from build123d import *

# Parameters (mm, degrees)
SKETCH1_R           = 2.5
BOSS_EXTRUDE3_DEPTH = 1.5
FILLET1_R           = 2.5
SKETCH3_R           = 10
SKETCH3_R_2         = 2.5
BOSS_EXTRUDE4_DEPTH = 7


with BuildPart() as part:
    # Sketch1 → Boss-Extrude3 (new body)
    with BuildSketch(Plane(origin=(0, 0, 0), x_dir=(0, 0, -1), z_dir=(1, 0, 0))):
        with BuildLine():
            Line((-34.72862652, 4.35), (-33.15, 4.35))
            Line((-33.15, 4.35), (-33.15, -4.35))
            Line((-33.15, -4.35), (-34.72862652, -4.35))
            ThreePointArc((-34.72862652, -4.35), (-24.748737342, -24.748737342), (-4.35, -34.72862652))
            Line((-4.35, -34.72862652), (-4.35, -33.15))
            Line((-4.35, -33.15), (4.35, -33.15))
            Line((4.35, -33.15), (4.35, -34.72862652))
            ThreePointArc((4.35, -34.72862652), (24.748737342, -24.748737342), (34.72862652, -4.35))
            Line((34.72862652, -4.35), (33.15, -4.35))
            Line((33.15, -4.35), (33.15, 4.35))
            Line((33.15, 4.35), (34.72862652, 4.35))
            ThreePointArc((34.72862652, 4.35), (24.748737342, 24.748737342), (4.35, 34.72862652))
            Line((4.35, 34.72862652), (4.35, 33.15))
            Line((4.35, 33.15), (-4.35, 33.15))
            Line((-4.35, 33.15), (-4.35, 34.72862652))
            ThreePointArc((-4.35, 34.72862652), (-24.748737342, 24.748737342), (-34.72862652, 4.35))
        make_face()
        Circle(SKETCH1_R, mode=Mode.SUBTRACT)
        with BuildLine():
            Line((9.270248109, 3.75), (27.243118397, 3.75))
            ThreePointArc((27.243118397, 3.75), (19.17641557, 19.71078603), (3, 27.335873866))
            Line((3, 27.335873866), (3, 9.539392014))
            ThreePointArc((3, 9.539392014), (6.783731432, 7.347175502), (9.270248109, 3.75))
        make_face(mode=Mode.SUBTRACT)
        with BuildLine():
            Line((-3, 9.539392014), (-3, 27.335873866))
            ThreePointArc((-3, 27.335873866), (-19.709993452, 19.177230199), (-27.407799985, 2.25))
            Line((-27.407799985, 2.25), (-9.743587635, 2.25))
            ThreePointArc((-9.743587635, 2.25), (-7.340542585, 6.790908228), (-3, 9.539392014))
        make_face(mode=Mode.SUBTRACT)
        with BuildLine():
            Line((9.743587635, -2.25), (27.407799985, -2.25))
            ThreePointArc((27.407799985, -2.25), (20.230473673, -18.627343744), (4.5, -27.129319933))
            Line((4.5, -27.129319933), (4.5, -8.93028555))
            ThreePointArc((4.5, -8.93028555), (7.866161766, -6.174422974), (9.743587635, -2.25))
        make_face(mode=Mode.SUBTRACT)
        with BuildLine():
            Line((-1.5, -9.886859967), (-1.5, -27.459060435))
            ThreePointArc((-1.5, -27.459060435), (-18.629857769, -20.22815858), (-27.243118397, -3.75))
            Line((-27.243118397, -3.75), (-9.270248109, -3.75))
            ThreePointArc((-9.270248109, -3.75), (-6.197969316, -7.847622338), (-1.5, -9.886859967))
        make_face(mode=Mode.SUBTRACT)
    extrude(amount=BOSS_EXTRUDE3_DEPTH)

    # Fillet1
    fillet1_edges = [part.edges().sort_by_distance(p)[0] for p in [
        (0.75, -9.886859967, 1.5),
        (0.75, -3.75, 9.270248109),
        (0.75, -3.75, 27.243118397),
        (0.75, -27.459060435, 1.5),
        (0.75, 27.335873866, 3),
        (0.75, 2.25, 27.407799985),
        (0.75, 2.25, 9.743587635),
        (0.75, 9.539392014, 3),
        (0.75, 3.75, -27.243118397),
        (0.75, 27.335873866, -3),
        (0.75, 9.539392014, -3),
        (0.75, 3.75, -9.270248109),
        (0.75, -2.25, -9.743587635),
        (0.75, -8.93028555, -4.5),
        (0.75, -27.129319933, -4.5),
        (0.75, -2.25, -27.407799985),
    ]]
    fillet(fillet1_edges, radius=FILLET1_R)

    # Sketch3 → Boss-Extrude4 (add)
    with BuildSketch(Plane(origin=(1.5, 0, 0), x_dir=(0, 0, -1), z_dir=(1, 0, 0))):
        with Locations(Location((0, 0, 0), (0, 0, 157.666317342))):
            Circle(SKETCH3_R)
        Circle(SKETCH3_R_2, mode=Mode.SUBTRACT)
    extrude(amount=BOSS_EXTRUDE4_DEPTH)


solid = part.part
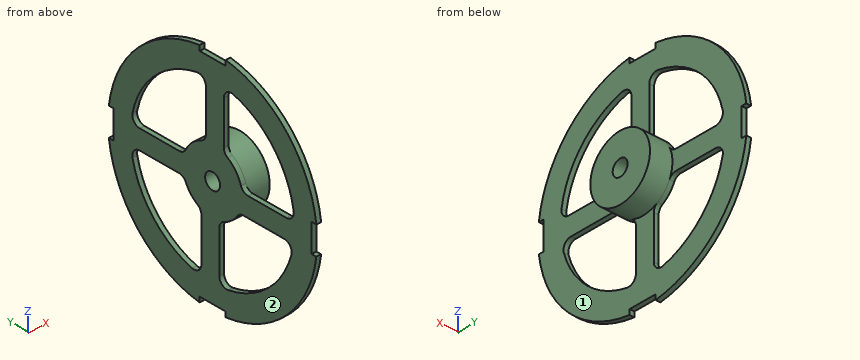
Geometry: final body of the model. Coordinates: model frame, mm. Face numbers are marked on the shaded views. A direction names the side the tool comes from. Coordinates: 2 decimals unless noted, no trailing zeros. Order: outer loops, then holes, each group sorted by start corner. A loop starts at its lowest first (then second) coordinate and runs counter-clockwise, first axis right, second up. Notation, with made-up numbers: (13, -38) - (51, -38) arc R21 ccw to (51, -2) - close; hole circle Ø3 at (36.25, 20.25). An arc over 180 degrees is marked (long way). Use one line per item in the form item = value.
1) Section D-D (z = -14). Return loops of the section in (x, y), then the cut area to 3 significant figures.
Solutions:
outline = (0, -32.08) - (1.5, -32.08) - (1.5, -23.67) - (0, -23.67) - close; (0, -2.25) - (1.5, -2.25) - (1.5, 3.75) - (0, 3.75) - close; (0, 23.67) - (1.5, 23.67) - (1.5, 32.08) - (0, 32.08) - close
area = 34.2 mm^2
2) Section C-C (y = 14). Return loops of the section in (x, z).
Solutions:
outline = (0, -32.08) - (1.5, -32.08) - (1.5, -23.67) - (0, -23.67) - close; (0, -3) - (1.5, -3) - (1.5, 3) - (0, 3) - close; (0, 23.67) - (1.5, 23.67) - (1.5, 32.08) - (0, 32.08) - close
3) Pin query (flat end, axial travel): pin 1 (1.2 mm diameter, centred on x = 0.5, z = -1.5, fed in from -Y); pin 2 (1.2 mm diameter, centred on x = 0.5, z = -19, fed in from +Y); pin 3 (1 mm diameter, centred on x = 1.5, y = 27.5, fed in from +Z). Return the tip coordinate at first contact, or that it passes through.
Solutions:
pin_1 = -33.15
pin_2 = 29.77
pin_3 = 22.27
4) Section A-A (y = 0). Return loops of the section in (x, z), then the cut area to 3 significant figures.
Solutions:
outline = (0, -33.15) - (1.5, -33.15) - (1.5, -10) - (8.5, -10) - (8.5, -2.5) - (0, -2.5) - close; (0, 2.5) - (8.5, 2.5) - (8.5, 10) - (1.5, 10) - (1.5, 33.15) - (0, 33.15) - close
area = 197 mm^2
5) Set-up query: the marked faces 1 and 2. Return all of +Z, -Z, +X, -X, +Y, -Y with unobstructed straight access to the full face (end or side cutting, diameter ignored); none if empty.
Solutions:
face_1 = +X
face_2 = +Z, -Z, -X, +Y, -Y
6) Ray query, L1, parallel to Y at x = 3, z = 0; L2, parallel to Y at x = 0.5, z = 11; L3, parallel to Z at x = 1, y = 19. Return the intervals inside material, ascending.
Solutions:
L1 = -10 to -2.5, 2.5 to 10
L2 = -33.23 to -25.2, -3.75 to 2.31, 25.2 to 33.23
L3 = -29.39 to -19.88, -3 to 3, 19.88 to 29.39
